Part model, mm, in its own coordinate system. A direction names the side the tool comes from. Round coordinates to 2 decimals unless told otherwise and drop trailing zeros. Loops run counter-clockwise (first coordinate to the right, second up) from the corner with the lowest first, then second, coordinate; pieces in that order, holes last.
from build123d import *

# Parameters (mm, degrees)
SALIENTE_EXTRUIR1_DEPTH = 48
CROQUIS2_R              = 1.5
CORTAR_EXTRUIR1_DEPTH   = 10
CORTAR_EXTRUIR2_START   = -38
CROQUIS2_2_R            = 1.5
CORTAR_EXTRUIR2_DEPTH   = 10


with BuildPart() as part:
    # Croquis1 → Saliente-Extruir1 (new body)
    with BuildSketch(Plane(origin=(0, 0, 0), x_dir=(1, 0, 0), z_dir=(0, 1, 0))):
        Polygon((0, 3.666174209), (-3.175, 1.833087105), (-3.175, -1.833087105), (0, -3.666174209), (3.175, -1.833087105), (3.175, 1.833087105), align=None)
    extrude(amount=SALIENTE_EXTRUIR1_DEPTH)

    # Croquis2 → Cortar-Extruir1 (cut)
    with BuildSketch(Plane(origin=(0, 48, 0), x_dir=(1, 0, 0), z_dir=(0, 1, 0))):
        with Locations(Location((0, 0, 0), (0, 0, 270))):
            Circle(CROQUIS2_R)
    extrude(amount=-CORTAR_EXTRUIR1_DEPTH, mode=Mode.SUBTRACT)

    # Croquis2_2 → Cortar-Extruir2 (cut)
    with BuildSketch(Plane(origin=(0, 48, 0), x_dir=(1, 0, 0), z_dir=(0, 1, 0)).offset(CORTAR_EXTRUIR2_START)):
        with Locations(Location((0, 0, 0), (0, 0, 270))):
            Circle(CROQUIS2_2_R)
    extrude(amount=-CORTAR_EXTRUIR2_DEPTH, mode=Mode.SUBTRACT)


solid = part.part
1) Drop flat-ended pins along their axis: pin 1 Ø1.5 at (x, y) = (-2.5, 8) entering from +Z; pin 2 Ø2.5 at (x, z) = (0, 0) entering from +Y; pin 3 Ø2 at (x, y) = (2.5, 10.5) entering from +Z. Give the stop position or say it passes through.
Values:
pin 1: stops at z = 2.66
pin 2: stops at y = 38
pin 3: stops at z = 2.8
2) Mould opens along X. For faces 1 (the face through (-1.57, 23.66, -2.76)), 2 (the face through (0, 0, 2)), 3 (the face through (0, 10, 0)) say: released by +X, released by -X, zero draft, split by the parting line, or undercut.
Values:
face 1: released by -X
face 2: zero draft
face 3: undercut
3) Tool access for faces 4 (the face through (0.45, 5.07, 1.43)), 5 (the face through (0, 38, 0)), 6 (the face through (0, 48, 2)): list every direction of +Z, -Z, +X, -X, +Y, -Y with a clear straight run to the whole face (end or side of a thin tool).
Values:
face 4: -Y
face 5: +Y
face 6: +Z, -Z, +X, -X, +Y
4) Wall check: line 1 along X through (y, z) = (45.5, 0) (3 decimals); line 2 along Y through (x, z) = (0, 1); line 3 along Z through (x, y) = (0.25, 38.5). Give the ranges that are in metal, low to high.
Values:
line 1: x = -3.175 to -1.5, 1.5 to 3.175
line 2: y = 10 to 38
line 3: z = -3.52 to -1.48, 1.48 to 3.52
5) Slice it at D-D, the plane z = 2.75. Give the cut face in (x, y).
Values:
outline: (-1.59, 0) - (1.59, 0) - (1.59, 48) - (-1.59, 48) - close
6) Slice it at A-A, the plane y = 7. Give the cut face in (x, z) (3 decimals).
Values:
outline: (-3.175, -1.833) - (0, -3.666) - (3.175, -1.833) - (3.175, 1.833) - (0, 3.666) - (-3.175, 1.833) - close; hole circle Ø3 at (0, 0)
7) Slice it at B-B, the plane z = 0. Give the cut face in (x, y) (3 decimals).
Values:
outline: (-3.175, 0) - (-1.5, 0) - (-1.5, 10) - (1.5, 10) - (1.5, 0) - (3.175, 0) - (3.175, 48) - (1.5, 48) - (1.5, 38) - (-1.5, 38) - (-1.5, 48) - (-3.175, 48) - close
8) Slice it at C-C, the plane y = 16. Give the cut face in (x, z) (3 decimals), then the cut area to 3 significant figures.
Values:
outline: (-3.175, -1.833) - (0, -3.666) - (3.175, -1.833) - (3.175, 1.833) - (0, 3.666) - (-3.175, 1.833) - close
area: 34.9 mm2
